For this review, take the finished solid that the model builds, in its own axes (mm). Give positions to 0.01 mm unless a question says otherwise; leave off trailing zeros. Order: outer loops, then holes, each group sorted by start corner. A loop starts at its lowest first (then second) coordinate and runs counter-clockwise, first axis right, second up. Notation, with made-up numbers: (81, -27) -> (109, -27) arc R17 ccw to (109, 5) -> close; hole circle Ø8 at (25.25, -27.5). An arc over 180 degrees is marked (long way). Use CSV: the item, a comma, the result in double quotes. Start each with the question number.
```python
from build123d import *

# Parameters (mm, degrees)
SKETCH1_W           = 63.5
SKETCH1_H           = 63.5
BOSS_EXTRUDE1_DEPTH = 3.175
SKETCH2_R           = 3.175
SKETCH2_R_2         = 7.9375
SKETCH2_R_3         = 2.38125
CUT_EXTRUDE1_DEPTH  = 4.175


with BuildPart() as part:
    # Sketch1 → Boss-Extrude1 (new body)
    with BuildSketch(Plane(origin=(0, 0, 0), x_dir=(1, 0, 0), z_dir=(0, 1, 0))):
        Rectangle(SKETCH1_W, SKETCH1_H)
    extrude(amount=BOSS_EXTRUDE1_DEPTH)

    # Sketch2 → Cut-Extrude1 (cut, through all)
    with BuildSketch(Plane(origin=(0, 3.175, 0), x_dir=(1, 0, 0), z_dir=(0, 1, 0))):
        with Locations((11.313708499, 11.313708499)):
            Circle(SKETCH2_R)
        with Locations((11.313708499, -11.313708499)):
            Circle(SKETCH2_R)
        with Locations((-11.313708499, -11.313708499)):
            Circle(SKETCH2_R)
        with Locations((-11.313708499, 11.313708499)):
            Circle(SKETCH2_R)
        Circle(SKETCH2_R_2)
        with Locations((-21.75, -21.75)):
            Circle(SKETCH2_R_3)
        with Locations((21.75, -21.75)):
            Circle(SKETCH2_R_3)
        with Locations((21.75, 21.75)):
            Circle(SKETCH2_R_3)
        with Locations((-21.75, 21.75)):
            Circle(SKETCH2_R_3)
    extrude(amount=-CUT_EXTRUDE1_DEPTH, mode=Mode.SUBTRACT)


solid = part.part
```
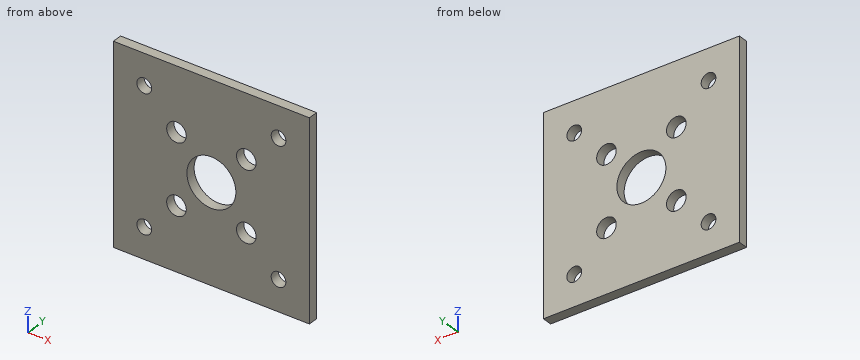
1. Consider section B-B (x = -21.75). State the section outline as (y, z) points (3 decimals).
2. Consider section C-C (z = 21.75). State the section outline as (x, y) points (3 decimals).
3. Consider section D-D (y = 2.1). State how many separate pieces and enclosed holes the cut face has, plus the area to 3 significant figures.
4. Clearance check with a flat-ended pin moving along its axis: P1, Ø7.5, axis at x = -11.31, z = -11.31, coming from the +Y side (3 decimals). State where the tip first meets the part, or that it passes through.
5. To check wall thickness, follow L1, parallel to Z at x = -21.75, y = 2.25; L2, parallel to X at y = 1.9, z = -11; L3, parallel to Z at x = 9, y = 2.2. State the ranges of each line that lie inside material, in increasing order. Write a range as [from, to].
Answer list:
1,outline,"(0, -31.75) -> (3.175, -31.75) -> (3.175, -24.131) -> (0, -24.131) -> close; (0, -19.369) -> (3.175, -19.369) -> (3.175, 19.369) -> (0, 19.369) -> close; (0, 24.131) -> (3.175, 24.131) -> (3.175, 31.75) -> (0, 31.75) -> close"
2,outline,"(-31.75, 0) -> (-24.131, 0) -> (-24.131, 3.175) -> (-31.75, 3.175) -> close; (-19.369, 0) -> (19.369, 0) -> (19.369, 3.175) -> (-19.369, 3.175) -> close; (24.131, 0) -> (31.75, 0) -> (31.75, 3.175) -> (24.131, 3.175) -> close"
3,separate pieces,"1"
3,enclosed holes,"9"
3,area,"3,640 mm2"
4,P1,"y = 3.175"
5,L1,"[-31.75, -24.13], [-19.37, 19.37], [24.13, 31.75]"
5,L2,"[-31.75, -14.47], [-8.15, 8.15], [14.47, 31.75]"
5,L3,"[-31.75, -13.49], [-9.14, 9.14], [13.49, 31.75]"
